Can you work these out from the model? Positions are in its coordinate system, mm. Give positions to 0.01 mm unless a question says otherwise; leave off trailing zeros. Order: outer loops, then holes, each group sorted by start corner. A loop starts at its lowest first (then second) coordinate and runs counter-clockwise, first axis right, second up. Notation, with made-up numbers: M 84.5,11 L 104.5,11 A24 cw 104.5,26 Z; hole C 34.5,35 d7. An arc over 180 degrees is marked long. Use one line per item in the form item = value. Start each with the question number.
1. Will these pins go through, and if not, where does the flat tip stop? P1, Ø4, axis at x = 36, y = -34, coming from the -Z side; P2, Ø4, axis at y = -19, z = 10.5, coming from the +X side; P3, Ø8, axis at x = 15.5, z = 20, coming from the +Y side.
2. I want a section at A-A, the plane z = 20.5. Count the separate pieces of the cut face and the enclosed holes in it, and give its area (3 significant figures).
3. I want a section at B-B, the plane y = 0. List the corners of the cut face in (x, z) for me.
4. I need wall thicknesses on L1, parallel to Y at x = 1, z = 15.25; L2, parallel to X at y = 34, z = 19; L3, parallel to Y at x = 36, z = 12.5. Which ranges of each line are inside material? Lowest first, please.
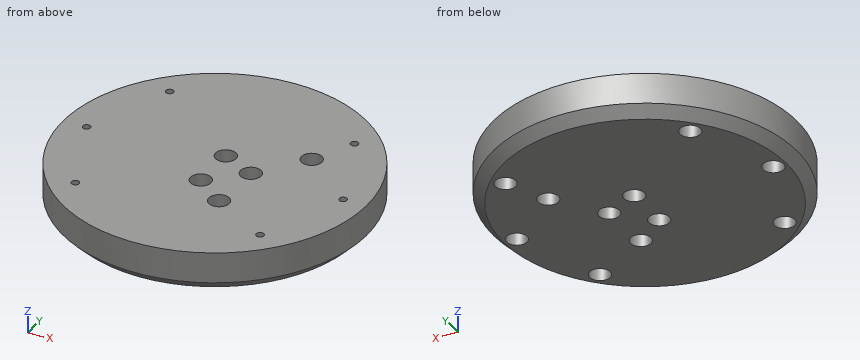
```python
from build123d import *

# Parameters (mm, degrees)
CYLINDER1536_R     = 4
CYLINDER1536_DEPTH = 100
CYLINDER1535_R     = 4
CYLINDER1535_DEPTH = 100
CYLINDER1484_R     = 1.5
CYLINDER1484_DEPTH = 100
CYLINDER1485_R     = 1.5
CYLINDER1485_DEPTH = 100
CYLINDER1486_R     = 1.5
CYLINDER1486_DEPTH = 100
CYLINDER1487_R     = 1.5
CYLINDER1487_DEPTH = 100
CYLINDER1488_R     = 1.5
CYLINDER1488_DEPTH = 100
CYLINDER1483_R     = 1.5
CYLINDER1483_DEPTH = 100
CYLINDER1133_R     = 4
CYLINDER1133_DEPTH = 100
CYLINDER1134_R     = 4
CYLINDER1134_DEPTH = 100
CYLINDER1135_R     = 4
CYLINDER1135_DEPTH = 100
CYLINDER1131_R     = 4
CYLINDER1131_DEPTH = 100
CYLINDER1136_R     = 4
CYLINDER1136_DEPTH = 100
CYLINDER1132_R     = 4
CYLINDER1132_DEPTH = 100
CYLINDER1508_R     = 4
CYLINDER1508_DEPTH = 20
CYLINDER1509_R     = 4
CYLINDER1509_DEPTH = 20
CYLINDER1510_R     = 4
CYLINDER1510_DEPTH = 20
CYLINDER1511_R     = 4
CYLINDER1511_DEPTH = 40
CYLINDER1512_R     = 4
CYLINDER1512_DEPTH = 40
CYLINDER1513_R     = 4
CYLINDER1513_DEPTH = 40
CYLINDER1514_R     = 4
CYLINDER1514_DEPTH = 40
CYLINDER1507_R     = 4
CYLINDER1507_DEPTH = 20
CYLINDER1489_R     = 59
CYLINDER1489_DEPTH = 16
CHAMFER040_SIZE    = 4


with BuildPart() as obj1:
    # Cylinder1536 → Cylinder1536 (new body)
    with BuildSketch(Plane(origin=(14, 0, -18), x_dir=(1, 0, 0), z_dir=(0, 0, 1))):
        Circle(CYLINDER1536_R)
    extrude(amount=CYLINDER1536_DEPTH)


with BuildPart() as obj2:
    # Cylinder1535 → Cylinder1535 (new body)
    with BuildSketch(Plane(origin=(90, 0, -18), x_dir=(1, 0, 0), z_dir=(0, 0, 1))):
        Circle(CYLINDER1535_R)
    extrude(amount=CYLINDER1535_DEPTH)

    # Compound905: union obj1
    add(obj1.part)


with BuildPart() as obj3:
    # Cylinder1484 → Cylinder1484 (new body)
    with BuildSketch(Plane(origin=(-36, 34, -60), x_dir=(1, 0, 0), z_dir=(0, 0, 1))):
        Circle(CYLINDER1484_R)
    extrude(amount=CYLINDER1484_DEPTH)


with BuildPart() as obj4:
    # Cylinder1485 → Cylinder1485 (new body)
    with BuildSketch(Plane(origin=(-36, -34, -60), x_dir=(1, 0, 0), z_dir=(0, 0, 1))):
        Circle(CYLINDER1485_R)
    extrude(amount=CYLINDER1485_DEPTH)


with BuildPart() as obj5:
    # Cylinder1486 → Cylinder1486 (new body)
    with BuildSketch(Plane(origin=(50, 0, -60), x_dir=(1, 0, 0), z_dir=(0, 0, 1))):
        Circle(CYLINDER1486_R)
    extrude(amount=CYLINDER1486_DEPTH)


with BuildPart() as obj6:
    # Cylinder1487 → Cylinder1487 (new body)
    with BuildSketch(Plane(origin=(36, 34, -60), x_dir=(1, 0, 0), z_dir=(0, 0, 1))):
        Circle(CYLINDER1487_R)
    extrude(amount=CYLINDER1487_DEPTH)


with BuildPart() as obj7:
    # Cylinder1488 → Cylinder1488 (new body)
    with BuildSketch(Plane(origin=(36, -34, -60), x_dir=(1, 0, 0), z_dir=(0, 0, 1))):
        Circle(CYLINDER1488_R)
    extrude(amount=CYLINDER1488_DEPTH)


with BuildPart() as obj8:
    # Cylinder1483 → Cylinder1483 (new body)
    with BuildSketch(Plane(origin=(-50, 0, -60), x_dir=(1, 0, 0), z_dir=(0, 0, 1))):
        Circle(CYLINDER1483_R)
    extrude(amount=CYLINDER1483_DEPTH)

    # Compound892: union obj3, obj4, obj5, obj6, obj7
    add(obj3.part)
    add(obj4.part)
    add(obj5.part)
    add(obj6.part)
    add(obj7.part)


with BuildPart() as obj9:
    # Cylinder1133 → Cylinder1133 (new body)
    with BuildSketch(Plane(origin=(-36, 34, -90), x_dir=(1, 0, 0), z_dir=(0, 0, 1))):
        Circle(CYLINDER1133_R)
    extrude(amount=CYLINDER1133_DEPTH)


with BuildPart() as obj10:
    # Cylinder1134 → Cylinder1134 (new body)
    with BuildSketch(Plane(origin=(-36, -34, -90), x_dir=(1, 0, 0), z_dir=(0, 0, 1))):
        Circle(CYLINDER1134_R)
    extrude(amount=CYLINDER1134_DEPTH)


with BuildPart() as obj11:
    # Cylinder1135 → Cylinder1135 (new body)
    with BuildSketch(Plane(origin=(50, 0, -90), x_dir=(1, 0, 0), z_dir=(0, 0, 1))):
        Circle(CYLINDER1135_R)
    extrude(amount=CYLINDER1135_DEPTH)


with BuildPart() as obj12:
    # Cylinder1131 → Cylinder1131 (new body)
    with BuildSketch(Plane(origin=(36, 34, -90), x_dir=(1, 0, 0), z_dir=(0, 0, 1))):
        Circle(CYLINDER1131_R)
    extrude(amount=CYLINDER1131_DEPTH)


with BuildPart() as obj13:
    # Cylinder1136 → Cylinder1136 (new body)
    with BuildSketch(Plane(origin=(36, -34, -90), x_dir=(1, 0, 0), z_dir=(0, 0, 1))):
        Circle(CYLINDER1136_R)
    extrude(amount=CYLINDER1136_DEPTH)


with BuildPart() as obj14:
    # Cylinder1132 → Cylinder1132 (new body)
    with BuildSketch(Plane(origin=(-50, 0, -90), x_dir=(1, 0, 0), z_dir=(0, 0, 1))):
        Circle(CYLINDER1132_R)
    extrude(amount=CYLINDER1132_DEPTH)

    # Compound897: union obj9, obj10, obj11, obj12, obj13
    add(obj9.part)
    add(obj10.part)
    add(obj11.part)
    add(obj12.part)
    add(obj13.part)


with BuildPart() as obj15:
    # Cylinder1508 → Cylinder1508 (new body)
    with BuildSketch(Plane(origin=(103, 6, -20), x_dir=(1, 0, 0), z_dir=(0, 0, 1))):
        Circle(CYLINDER1508_R)
    extrude(amount=CYLINDER1508_DEPTH)


with BuildPart() as obj16:
    # Cylinder1509 → Cylinder1509 (new body)
    with BuildSketch(Plane(origin=(76, 18, -18), x_dir=(1, 0, 0), z_dir=(0, 0, 1))):
        Circle(CYLINDER1509_R)
    extrude(amount=CYLINDER1509_DEPTH)


with BuildPart() as obj17:
    # Cylinder1510 → Cylinder1510 (new body)
    with BuildSketch(Plane(origin=(91, -21, -18), x_dir=(1, 0, 0), z_dir=(0, 0, 1))):
        Circle(CYLINDER1510_R)
    extrude(amount=CYLINDER1510_DEPTH)


with BuildPart() as obj18:
    # Cylinder1511 → Cylinder1511 (new body)
    with BuildSketch(Plane(origin=(13, -21, -18), x_dir=(1, 0, 0), z_dir=(0, 0, 1))):
        Circle(CYLINDER1511_R)
    extrude(amount=CYLINDER1511_DEPTH)


with BuildPart() as obj19:
    # Cylinder1512 → Cylinder1512 (new body)
    with BuildSketch(Plane(origin=(28, 18, -18), x_dir=(1, 0, 0), z_dir=(0, 0, 1))):
        Circle(CYLINDER1512_R)
    extrude(amount=CYLINDER1512_DEPTH)


with BuildPart() as obj20:
    # Cylinder1513 → Cylinder1513 (new body)
    with BuildSketch(Plane(origin=(1, -12, -18), x_dir=(1, 0, 0), z_dir=(0, 0, 1))):
        Circle(CYLINDER1513_R)
    extrude(amount=CYLINDER1513_DEPTH)


with BuildPart() as obj21:
    # Cylinder1514 → Cylinder1514 (new body)
    with BuildSketch(Plane(origin=(1, 6, -18), x_dir=(1, 0, 0), z_dir=(0, 0, 1))):
        Circle(CYLINDER1514_R)
    extrude(amount=CYLINDER1514_DEPTH)


with BuildPart() as obj22:
    # Cylinder1507 → Cylinder1507 (new body)
    with BuildSketch(Plane(origin=(103, -12, -20), x_dir=(1, 0, 0), z_dir=(0, 0, 1))):
        Circle(CYLINDER1507_R)
    extrude(amount=CYLINDER1507_DEPTH)

    # Compound895: union obj15, obj16, obj17, obj18, obj19, obj20, obj21
    add(obj15.part)
    add(obj16.part)
    add(obj17.part)
    add(obj18.part)
    add(obj19.part)
    add(obj20.part)
    add(obj21.part)


with BuildPart() as cut529:
    # Cylinder1489 → Cylinder1489 (new body)
    with BuildSketch(Plane.XY.offset(2)):
        Circle(CYLINDER1489_R)
    extrude(amount=CYLINDER1489_DEPTH)

    # Cut512: cut obj22
    add(obj22.part, mode=Mode.SUBTRACT)

    # Cut516: cut obj14
    add(obj14.part, mode=Mode.SUBTRACT)

    # Cut518: cut obj8
    add(obj8.part, mode=Mode.SUBTRACT)

    # Chamfer040
    chamfer040_edges = [cut529.edges().sort_by_distance(p)[0] for p in [
        (-59, 0, 2),
    ]]
    chamfer(chamfer040_edges, length=CHAMFER040_SIZE)

    # Cut529: cut obj2
    add(obj2.part, mode=Mode.SUBTRACT)


with BuildPart() as cut529_1:
    # Cut529 placement: moved
    add(cut529.part.moved(Location((0, 0, 4))))


solid = cut529_1.part
```
Check result:
q1.P1 = 14
q1.P2 = 56.5
q1.P3 = 57.87
q2.separate_pieces = 1
q2.enclosed_holes = 11
q2.area = 10,600 mm2
q3.outline = M -59,10 L -55,6 L -54,6 L -54,14 L -51.5,14 L -51.5,22 L -59,22 Z; M -48.5,14 L -46,14 L -46,6 L 10,6 L 10,22 L -48.5,22 Z; M 18,6 L 46,6 L 46,14 L 48.5,14 L 48.5,22 L 18,22 Z; M 51.5,14 L 54,14 L 54,6 L 55,6 L 59,10 L 59,22 L 51.5,22 Z
q4.L1 = -58.99 to -16, -8 to 2, 10 to 58.99
q4.L2 = -48.22 to -37.5, -34.5 to 34.5, 37.5 to 48.22
q4.L3 = -46.74 to -38, -30 to 30, 38 to 46.74
